from build123d import *

# Parameters (mm, degrees)
F0_R     = 3
F1_DEPTH = 5
F2_W     = 40
F2_H     = 11
F3_DEPTH = 25
F5_DEPTH = 11.001
F7_DEPTH = 25


with BuildPart() as f1:
    # F0 (on Top) → F1 (new body, symmetric)
    with BuildSketch(Plane.XY):
        Circle(F0_R)
    extrude(amount=F1_DEPTH, both=True)

    # F2 (on Front) → F3 (join)
    with BuildSketch(Plane.XZ):
        with Locations((0.3750487044, 5.5)):
            Rectangle(F2_W, F2_H)
    extrude(amount=F3_DEPTH)

    # F4 (on Top) → F5 (cut, through all)
    with BuildSketch(Plane.XY):
        Polygon((-19.9439544231, -25.4493262619), (-3.0048058834, 0), (-26.9990675151, 2.6770541444), align=None)
        Polygon((32.6401479542, 2.6770541444), (3.0086771585, 0), (20.6934921443, -25.4493262619), align=None)
    extrude(amount=F5_DEPTH, mode=Mode.SUBTRACT)


with BuildPart() as f7:
    # F6 (on Right) → F7 (new body, symmetric)
    with BuildSketch(Plane.YZ):
        Polygon((6.2013822608, 13.6782731861), (-25.7219970226, 11.1731654033), (6.2013822608, 3.444124246), align=None)
    extrude(amount=F7_DEPTH, both=True)


with BuildPart() as f1_1:
    add(f1.part)

    # F8: cut F7
    add(f7.part, mode=Mode.SUBTRACT)


solid = f1_1.part
The model under review builds one solid part; all positions refer to its coordinate system, in mm. A direction names the side the tool comes from. Round coordinates to 2 decimals unless told otherwise and drop trailing zeros. Write each loop counter-clockwise with the first axis right and the second up, starting at its lowest first coordinate (ties: lowest second). Pieces come first, ordered by that corner, then holes. Notation, with made-up numbers: M 55,40.5 L 87,40.5 A16 cw 87,55.5 Z; hole C -14,87.5 d6. An arc over 180 degrees is marked long. Answer as CSV lines item,"result". Start each with the question number.
Q1. Wall thickness on line 1 along Z through (x, y) = (11.5, -19.5); line 2 along Z through (x, y) = (-15, -22.25); line 3 along Y through (x, z) = (-15.5, 8): over which ranges is each line inside the solid? List them lowest first.
Q2. Consider section A-A, the plane x = 0. Give the boundary of the cut face in (y, z), then the cut area to 3 significant figures.
Q3. Clearance check with flat-ended pins moving along their axes: P1, Ø10, axis at x = -11, y = -10.5, coming from the +Z side; P2, Ø4, axis at x = -7.5, y = -7.5, coming from the -Z side; P3, Ø1.5, axis at x = 1.5, z = -1, coming from the +Y side. State where each tip first meets the part, or that it passes through.
Q4. Consider section B-B, the plane z = -3.25. Give the boundary of the cut face in (x, y).
Q5. Consider section C-C, the plane y = -4.75. Give the boundary of the cut face in (x, z).
Q6. Tool access review of faces 1 (the face through (0, 3, -1)), 2 (the face through (0, 0, -5)): name each direction out of +Z, -Z, +X, -X, +Y, -Y from which nothing blocks a thin tool from reaching the whole face with its end or side.
Result set:
1,line 1,"z = 0 to 9.67"
1,line 2,"z = 0 to 10.33"
1,line 3,"y = -25 to -18.77"
2,outline,"M -25,0 L -3,0 L -3,-5 L 3,-5 L 3,4.22 L -25,11 Z"
2,area,"243 mm²"
3,P1,"stops at z = 8.7"
3,P2,"stops at z = 0"
3,P3,"stops at y = 2.9"
4,outline,"C 0,0 d6"
5,outline,"M -6.17,0 L 6.31,0 L 6.31,6.1 L -6.17,6.1 Z"
6,face 1,"-Z"
6,face 2,"-Z, +X, -X, +Y, -Y"
